from build123d import *

# Parameters (mm, degrees)
SKETCH1_R           = 2.75
BOSS_EXTRUDE1_DEPTH = 3
CUT_EXTRUDE1_DEPTH  = 1.3
SKETCH9_R           = 1.5
BOSS_EXTRUDE2_DEPTH = 12
CHAMFER1_SIZE       = 0.2805
FILLET1_R           = 0.1


with BuildPart() as part:
    # Sketch1 → Boss-Extrude1 (new body)
    with BuildSketch(Plane(origin=(0, 0, 0), x_dir=(0, -1, 0), z_dir=(-1, 0, 0))):
        Circle(SKETCH1_R)
    extrude(amount=-BOSS_EXTRUDE1_DEPTH)

    # Sketch2 → Cut-Extrude1 (cut)
    with BuildSketch(Plane.ZY):
        Polygon((0, -1.478016689), (1.28, -0.739008345), (1.28, 0.739008345), (0, 1.478016689), (-1.28, 0.739008345), (-1.28, -0.739008345), align=None)
    extrude(amount=-CUT_EXTRUDE1_DEPTH, mode=Mode.SUBTRACT)

    # Sketch4 → Cut-Revolve1 (revolve, cut)
    with BuildSketch(Plane.XY):
        Polygon((1.3, 1.28), (1.3, 0), (2.039008345, 0), align=None)
    revolve(axis=Axis((1.3, 0, 0), (1, 0, 0)), mode=Mode.SUBTRACT)

    # Sketch9 → Boss-Extrude2 (add)
    with BuildSketch(Plane(origin=(3, 0, 0), x_dir=(0, 0, -1), z_dir=(1, 0, 0))):
        Circle(SKETCH9_R)
    extrude(amount=BOSS_EXTRUDE2_DEPTH)

    # Chamfer1
    chamfer1_edges = [part.edges().sort_by_distance(p)[0] for p in [
        (0, 2.75, 0),
        (15, 0, 1.5),
    ]]
    chamfer(chamfer1_edges, length=CHAMFER1_SIZE)

    # Fillet1
    fillet1_edges = [part.edges().sort_by_distance(p)[0] for p in [
        (3, 0, 1.5),
    ]]
    fillet(fillet1_edges, radius=FILLET1_R)


solid = part.part
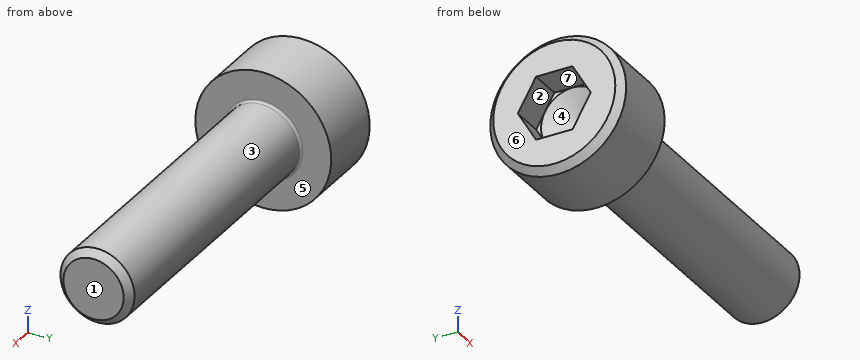
Can you work these out from the model? Positions are in its coordinate system, mm. Face numbers are marked on the shaded views. A direction names the side the tool comes from. Round coordinates to 2 decimals unless told otherwise and drop trailing zeros. Loops run counter-clockwise (first coordinate to the right, second up) from the corner with the lowest first, then second, coordinate; pieces in that order, holes last. Notation, with made-up numbers: (5.25, 17) - (46.25, 17) arc R22 cw to (46.25, 52) - close; hole circle Ø6 at (-17, 52.5). An arc over 180 degrees is marked (long way). Write item = value, one per line. Start each with the question number.
(1) If we section it at A-A (x = 7.75): Please give me the cut outline in (y, z).
(2) If we mould it in two halves opening along Z, with no side actions, what happens to the marked faces 1, 2, 3 and 4? For each: released by +Z, released by -Z, zero draft, split by the parting line, or undercut.
(3) For P1, Ø0.5, axis at y = -0.5, z = 1, coming from the -X side; P2, Ø1.5, axis at x = 6, y = 1.5, coming from the +Z side; P3, Ø2, axis at x = 10.5, z = 2, coming from the +Y side, each with a flat end and sliding along its axis, tell me the tip position at first contact or that it passes through.
(4) If I drill on probe 1 along Z at (x, y) = (0.5, -0.1); probe 2 along X at (y, z) = (-0.55, 1.5); probe 3 along Z at (x, y) = (0.5, -1.2), over which ranges is the centre line in solid material (lowest first)? Write a range as [from, to].
(5) For the marked faces 5, 6 and 7, which set-ups out of +Z, -Z, +X, -X, +Y, -Y let a thin tool reach every point of the face, with its end or its side?
Ans:
q1.outline = circle Ø3 at (0, 0)
q2.face_1 = zero draft
q2.face_2 = undercut
q2.face_3 = split by the parting line
q2.face_4 = undercut
q3.P1 = 1.3
q3.P2 = 1.3
q3.P3 = 1.12
q4.probe_1 = [-2.75, -1.28], [1.28, 2.75]
q4.probe_2 = [0, 3]
q4.probe_3 = [-2.47, -0.48], [0.48, 2.47]
q5.face_5 = +X
q5.face_6 = +Z, -Z, -X, +Y, -Y
q5.face_7 = -X
